```python
from build123d import *

# Parameters (mm, degrees)
EXTRUDE_1_DEPTH     = 5
FILLET_1_R          = 5
SKETCH_7_R          = 1.75
CUT_EXTRUDE_5_DEPTH = 91.056926441
SKETCH_8_R          = 1.75
CUT_EXTRUDE_6_DEPTH = 91.056926441
SKETCH_9_R          = 1.75
SKETCH_9_R_2        = 2
CUT_EXTRUDE_7_DEPTH = 91.056926441


with BuildPart() as part:
    # 스케치2 → 보스-돌출1 (new body)
    with BuildSketch(Plane(origin=(0, 0, 0), x_dir=(1, 0, 0), z_dir=(0, 1, 0))):
        Polygon((-60, -25), (-60, -52.5), (-73, -52.5), (-73, 52.5), (-60, 52.5), (-60, 25), (0, 25), (0, -25), align=None)
    extrude(amount=EXTRUDE_1_DEPTH)

    # 필렛1
    fillet_1_edges = [part.edges().sort_by_distance(p)[0] for p in [
        (0, 2.5, 25),
        (-60, 2.5, 25),
        (-60, 2.5, 52.5),
        (-73, 2.5, 52.5),
        (-73, 2.5, -52.5),
        (-60, 2.5, -52.5),
        (-60, 2.5, -25),
        (0, 2.5, -25),
    ]]
    fillet(fillet_1_edges, radius=FILLET_1_R)

    # 스케치7 → 컷-돌출5 (cut, through all)
    with BuildSketch(Plane.XZ):
        with Locations(Location((-66.5, -46, 0), (0, 0, 270))):
            Circle(SKETCH_7_R)
        with Locations(Location((-66.5, 46, 0), (0, 0, 270))):
            Circle(SKETCH_7_R)
    extrude(amount=-CUT_EXTRUDE_5_DEPTH, mode=Mode.SUBTRACT)

    # 스케치8 → 컷-돌출6 (cut, through all)
    with BuildSketch(Plane(origin=(0, 5, 0), x_dir=(1, 0, 0), z_dir=(0, 1, 0))):
        with Locations(Location((-5, 20, 0), (0, 0, 270))):
            Circle(SKETCH_8_R)
        with Locations(Location((-5, -20, 0), (0, 0, 270))):
            Circle(SKETCH_8_R)
    extrude(amount=-CUT_EXTRUDE_6_DEPTH, mode=Mode.SUBTRACT)

    # 스케치9 → 컷-돌출7 (cut, through all)
    with BuildSketch(Plane(origin=(0, 5, 0), x_dir=(1, 0, 0), z_dir=(0, 1, 0))):
        with Locations(Location((-52, 18.5, 0), (0, 0, 270))):
            Circle(SKETCH_9_R)
        with Locations(Location((-52, -18.5, 0), (0, 0, 270))):
            Circle(SKETCH_9_R)
        with Locations(Location((-15, -18.5, 0), (0, 0, 270))):
            Circle(SKETCH_9_R)
        with Locations(Location((-15, 18.5, 0), (0, 0, 270))):
            Circle(SKETCH_9_R)
        with Locations(Location((-33.5, 20, 0), (0, 0, 270))):
            Circle(SKETCH_9_R_2)
        with Locations(Location((-33.5, -20, 0), (0, 0, 270))):
            Circle(SKETCH_9_R_2)
    extrude(amount=-CUT_EXTRUDE_7_DEPTH, mode=Mode.SUBTRACT)


solid = part.part
```
Geometry check sheet. Reference: the model listing, model coordinates, mm. A direction names the side the tool comes from. Coordinates: 2 decimals unless noted, no trailing zeros. Write each loop counter-clockwise with the first axis right and the second up, starting at its lowest first coordinate (ties: lowest second). Pieces come first, ordered by that corner, then holes. Notation, with made-up numbers: M 32.25,14.5 L 36.25,14.5 A28 cw 36.25,48.5 Z; hole C -13.5,37 d10. An arc over 180 degrees is marked long. Use one line per item in the form item = value. Start each with the question number.
1) Section check D-D on x = -33.5. Enter the section's corners in (y, z), and give its area (3 significant figures).
2) Section check B-B on z = -46. Enter the section's corners in (x, y), and give its area (3 significant figures).
3) Section check C-C on y = 2.4. State how many separate pieces and enclosed holes the cut face has, and give its area (3 significant figures).
4) Section check A-A on x = -15. Enter the section's corners in (y, z).
5) Go/stop test with flat-tipped pins: pin 1 Ø1.5 at (x, y) = (-54.5, 2.5) entering from +Z; pin 2 Ø2 at (x, z) = (-5, 20) entering from -Y. Record where each tip stops, or that it passes through.
6) Set-up check for faces 1 (the flat face through (-60, 2, 39)), 2 (the flat face through (-66, 2, 52.5)), 3 (the flat face through (-30, 2, -25)): record each of +Z, -Z, +X, -X, +Y, -Y from which the full face is reachable in a straight line by a thin tool's end or side.
7) Thickness scan on probe 1 along Z at (x, y) = (-66, 3.5); probe 2 along X at (y, z) = (2.75, 46); probe 3 along X at (y, z) = (1.3, -18.5). Record the ranges inside material, lowest first. Write a range as from..to.
Responses:
q1.outline = M 0,-25 L 5,-25 L 5,-22 L 0,-22 Z; M 0,-18 L 5,-18 L 5,18 L 0,18 Z; M 0,22 L 5,22 L 5,25 L 0,25 Z
q1.area = 210 mm2
q2.outline = M -73,0 L -68.25,0 L -68.25,5 L -73,5 Z; M -64.75,0 L -60,0 L -60,5 L -64.75,5 Z
q2.area = 47.5 mm2
q3.separate_pieces = 1
q3.enclosed_holes = 10
q3.area = 4,240 mm2
q4.outline = M 0,-25 L 5,-25 L 5,-20.25 L 0,-20.25 Z; M 0,-16.75 L 5,-16.75 L 5,16.75 L 0,16.75 Z; M 0,20.25 L 5,20.25 L 5,25 L 0,25 Z
q5.pin_1 = 25.01
q5.pin_2 = through
q6.face_1 = +Z, +X, +Y, -Y
q6.face_2 = +Z, +X, -X, +Y, -Y
q6.face_3 = -Z, +X, +Y, -Y
q7.probe_1 = -52.5..-47.68, -44.32..44.32, 47.68..52.5
q7.probe_2 = -73..-68.25, -64.75..-60
q7.probe_3 = -73..-53.75, -50.25..-34.82, -32.18..-16.75, -13.25..-5.9, -4.1..0
